For this review, take the finished solid that the model builds, in its own axes (mm). Give positions to 0.01 mm unless a question says otherwise; leave off trailing zeros. Loops run counter-clockwise (first coordinate to the right, second up) from the corner with the lowest first, then second, coordinate; pieces in that order, holes last. Notation, with made-up numbers: (48, 56) - (60, 56) arc R32 ccw to (60, 86) - close; hole circle Ø8 at (-11.75, -20.5). An arc over 180 degrees is marked (long way). Answer as CSV lines item,"result".
from build123d import *

# Parameters (mm, degrees)
SKETCH1_R           = 2.667
SKETCH1_R_2         = 2.2479
SKETCH1_R_3         = 3.429
BOSS_EXTRUDE1_DEPTH = 1.5875
SKETCH4_W           = 30.98284419
SKETCH4_H           = 26.473645648
CUT_EXTRUDE2_DEPTH  = 402.23458743
SKETCH5_W           = 76.2
SKETCH5_H           = 19.05
SKETCH5_W_2         = 19.05
SKETCH5_H_2         = 76.2
BOSS_EXTRUDE2_DEPTH = 1.27


with BuildPart() as part:
    # Sketch1 → Boss-Extrude1 (new, symmetric)
    with BuildSketch(Plane(origin=(0, 0, 0), x_dir=(1, 0, 0), z_dir=(0, 1, 0))):
        Polygon((-298.45, 13.124176698), (-298.45, 236.855), (298.45, 236.855), (298.45, 13.124176698), (323.85, 13.124176698), (323.85, -236.855), (-323.85, -236.855), (-323.85, 13.124176698), align=None)
        with Locations(Location((91.135199987, -18.161, 0), (0, 0, 270))):
            Circle(SKETCH1_R, mode=Mode.SUBTRACT)
        with Locations(Location((91.135199987, -122.555, 0), (0, 0, 270))):
            Circle(SKETCH1_R, mode=Mode.SUBTRACT)
        with Locations(Location((-91.135199987, -122.555, 0), (0, 0, 270))):
            Circle(SKETCH1_R, mode=Mode.SUBTRACT)
        with Locations(Location((-91.135199987, -18.161, 0), (0, 0, 270))):
            Circle(SKETCH1_R, mode=Mode.SUBTRACT)
        with Locations(Location((-295.275, -71.755, 0), (0, 0, 270))):
            Circle(SKETCH1_R_2, mode=Mode.SUBTRACT)
        with Locations(Location((-244.475, -71.755, 0), (0, 0, 270))):
            Circle(SKETCH1_R_2, mode=Mode.SUBTRACT)
        with Locations(Location((-244.475, -122.555, 0), (0, 0, 270))):
            Circle(SKETCH1_R_2, mode=Mode.SUBTRACT)
        with Locations(Location((-295.275, -122.555, 0), (0, 0, 270))):
            Circle(SKETCH1_R_2, mode=Mode.SUBTRACT)
        with Locations(Location((295.275, -122.555, 0), (0, 0, 90))):
            Circle(SKETCH1_R_2, mode=Mode.SUBTRACT)
        with Locations(Location((244.475, -122.555, 0), (0, 0, 90))):
            Circle(SKETCH1_R_2, mode=Mode.SUBTRACT)
        with Locations(Location((244.475, -71.755, 0), (0, 0, 90))):
            Circle(SKETCH1_R_2, mode=Mode.SUBTRACT)
        with Locations(Location((295.275, -71.755, 0), (0, 0, 90))):
            Circle(SKETCH1_R_2, mode=Mode.SUBTRACT)
        with Locations(Location((-193.675, -2.042328148, 0), (0, 0, 270))):
            Circle(SKETCH1_R_3, mode=Mode.SUBTRACT)
        with Locations(Location((-165.455833426, -59.055, 0), (0, 0, 270))):
            Circle(SKETCH1_R_3, mode=Mode.SUBTRACT)
    extrude(amount=BOSS_EXTRUDE1_DEPTH, both=True)

    # Sketch4 → Cut-Extrude2 (cut, through all)
    with BuildSketch(Plane(origin=(0, 1.5875, 0), x_dir=(1, 0, 0), z_dir=(0, 1, 0))):
        with Locations((0, -236.855)):
            Rectangle(SKETCH4_W, SKETCH4_H)
    extrude(amount=-CUT_EXTRUDE2_DEPTH, mode=Mode.SUBTRACT)

    # Sketch5 → Boss-Extrude2 (add)
    with BuildSketch(Plane(origin=(0, 1.5875, 0), x_dir=(1, 0, 0), z_dir=(0, 1, 0))):
        with Locations((0, 84.455)):
            Rectangle(SKETCH5_W, SKETCH5_H)
        with Locations((-79.375, 151.421322831)):
            Rectangle(SKETCH5_W_2, SKETCH5_H_2)
        with Locations((79.375, 151.421322831)):
            Rectangle(SKETCH5_W_2, SKETCH5_H_2)
        with Locations((171.623795352, -33.052997334)):
            Rectangle(SKETCH5_W_2, SKETCH5_H_2)
    extrude(amount=BOSS_EXTRUDE2_DEPTH)


solid = part.part
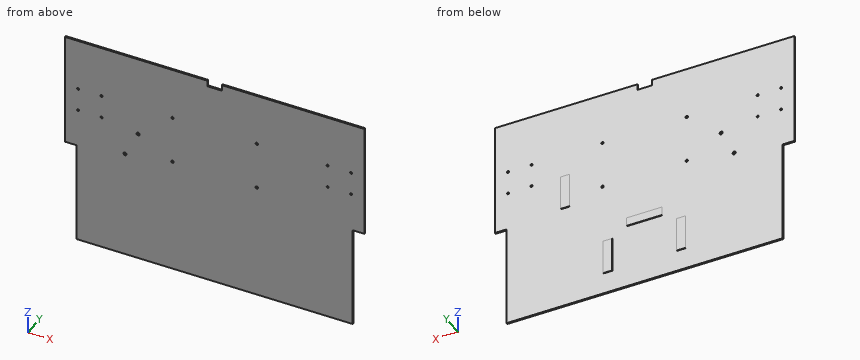
1) Consider section C-C on y = 0.3. Count the separate pieces of the cut face and the enclosed holes in it, and give its area (3 significant figures).
From the geometry:
separate pieces,"1"
enclosed holes,"14"
area,"295,000 mm^2"
2) Insertion check: P1, Ø0.6, axis at y = 2, z = -82.5, coming from the -X side; P2, Ø1.6, axis at y = -0.5, z = -109.5, coming from the +X side; P3, Ø8.5, axis at x = 91.14, z = 122.56, coming from the +Y side. Each pin has a flat end and moves straight along its axis. Give the tip position at first contact, or say it passes through.
From the geometry:
P1,"stops at x = -38.1"
P2,"stops at x = 298.45"
P3,"stops at y = 1.59"
3) Wall thickness on line 1 (X direction, y = 1.7, z = -181); line 2 (Y direction, x = -248, z = -104.5); line 3 (Z direction, x = 294, y = 0.65) (3 decimals): over which ranges is each line inside the solid? List them lowest first. Write a range as from..to.
From the geometry:
line 1,"x = -88.9..-69.85, 69.85..88.9"
line 2,"y = -1.59..1.59"
line 3,"z = -236.855..69.904, 73.606..120.704, 124.406..236.855"
4) Consider section B-B on z = -129. Write out the cut boundary in (x, y), and give its area (3 significant figures).
From the geometry:
outline,"(-298.45, -1.59) - (298.45, -1.59) - (298.45, 1.59) - (88.9, 1.59) - (88.9, 2.86) - (69.85, 2.86) - (69.85, 1.59) - (-69.85, 1.59) - (-69.85, 2.86) - (-88.9, 2.86) - (-88.9, 1.59) - (-298.45, 1.59) - close"
area,"1,940 mm^2"
5) Consider section A-A on x = -25. Write out the cut boundary in (y, z) (1 decimal), and give its area (3 significant figures).
From the geometry:
outline,"(-1.6, -236.9) - (1.6, -236.9) - (1.6, -94) - (2.9, -94) - (2.9, -74.9) - (1.6, -74.9) - (1.6, 236.9) - (-1.6, 236.9) - close"
area,"1,530 mm^2"
6) Consider section D-D on x = -113. Write out the cut boundary in (y, z) (1 decimal), and give its area (3 significant figures).
From the geometry:
outline,"(-1.6, -236.9) - (1.6, -236.9) - (1.6, 236.9) - (-1.6, 236.9) - close"
area,"1,500 mm^2"
